Could you check a few things on this model? Use its own coordinates, in mm. A direction names the side the tool comes from. Coordinates: 2 decimals unless noted, no trailing zeros. Order: outer loops, then holes, each group sorted by start corner. A loop starts at its lowest first (then second) coordinate and runs counter-clockwise, first axis right, second up. Notation, with made-up numbers: (22.5, 16) -> (44.5, 16) arc R18 ccw to (44.5, 22) -> close; hole circle Ø10 at (16, 56.25). An arc over 180 degrees is marked (long way). Use a Markdown table: item, result. Add a question column.
1) If we section it at D-D (x = -157): Write out the boundary of the cut face in (y, z), plus the area to 3 significant figures.
2) If I drill on L1, parallel to Z at x = -50, y = 1.6; L2, parallel to Z at x = -3, y = 2.5; L3, parallel to Z at x = -130, y = 4, over which ranges is the centre line in solid material (lowest first)? Write a range as [from, to].
3) If we section it at C-C (y = -53): Write out the boundary of the cut face in (x, z), plus the area to 3 significant figures.
4) Which directions (+Z, -Z, +X, -X, +Y, -Y) give clear straight access to the entire face, cutting with the end or side of a thin tool? Please do faces 1 (the flat face through (-125, 3, 174)), 2 (the flat face through (-89, 0, 98)), 3 (the flat face through (-89, 5, 101)).
5) Will these pins go through, and if not, where does the flat tip stop? pin 1 Ø3 at (x, y) = (-146.24, -11.72) entering from -Z; pin 2 Ø5.5 at (x, y) = (-146.24, -43.28) entering from -Z; pin 3 Ø1.6 at (y, z) = (3, 120) entering from +X; pin 4 Ø12 at (x, z) = (-144.5, 20) entering from -Y.
6) If we section it at B-B (z = 73.5): Write out the boundary of the cut face in (x, y).
7) If we section it at A-A (x = -50): Write out the boundary of the cut face in (y, z), plus the area to 3 significant figures.
8) Thinking about a two-plate mould opening in Z: for faces 4 (the flat face through (-89, -27, 200)), 5 (the flat face through (0, 2, 130)), 6 (the cylindrical face through (-23.02, 1.48, 80.69)), 7 (the cylindrical face through (-42.413, 3.986, 174.168)), which applies, +Z half, -Z half, draft (parallel to the pull), parting line (faces both ways), or undercut?
Autodesk Inventor part; units mm, degrees
ref_plane "YZ Plane" through (0, 0, 0) normal (1, 0, 0) x (0, 1, 0)
ref_plane "XZ Plane" through (0, 0, 0) normal (0, 1, 0) x (-1, 0, 0)
ref_plane "XY Plane" through (0, 0, 0) normal (0, 0, 1) x (1, 0, 0)
sketch "Sketch1" plane through (0, 0, 0) normal (0, 1, 0) x (-1, 0, 0)
  line L0 (0, 0) -> (180, 0)
  line L1 (180, 0) -> (180, 200)
  line L2 (180, 200) -> (0, 200)
  line L3 (0, 200) -> (0, 0)
  circle A0 centre (130, 140) radius 35
  circle A1 centre (130, 60) radius 35
  circle A2 centre (50, 140) radius 35
  circle A3 centre (50, 60) radius 35
  line L4 (130, 140) -> (50, 140)
  line L5 (130, 140) -> (130, 60)
  circle A4 centre (130, 140) radius 34
  circle A5 centre (130, 60) radius 34
  circle A6 centre (50, 140) radius 34
  circle A7 centre (50, 60) radius 34
  point P0 (90, 140)
  point P1 (90, 200)
  point P2 (130, 100)
  point P3 (180, 100)
  dimension "d0" = 180
  dimension "d1" = 200
  dimension "d2" = 70
  dimension "d3" = 70
  dimension "d4" = 70
  dimension "d5" = 70
  dimension "d6" = 10
  dimension "d7" = 10
  dimension "d11" = 68
  dimension "d12" = 68
  dimension "d13" = 68
  dimension "d14" = 68
extrude "Extrusion1" add sketch "Sketch1" along normal blind 5 contours L3 L2 L1 L0
extrude "Extrusion2" add sketch "Sketch1" along normal blind 3 contours A0 L5 A4 L4 | A1 | A2 | L4 A4 L5 A0 | A3
sketch "Sketch2" plane through (0, 0, 200) normal (1, 0, 0) x (0, 0, -1)
  circle A0 centre (40, 2.5) radius 1
  circle A1 centre (80, 2.5) radius 1
  circle A2 centre (120, 2.5) radius 1
  circle A3 centre (160, 2.5) radius 1
  line L0 (0, 0) -> (0, 5)
  line L1 (200, 0) -> (200, 5)
  line L2 (0, 5) -> (200, 5)
  dimension "d18" = 2
  dimension "d19" = 2
  dimension "d20" = 2
  dimension "d21" = 2
  dimension "d23" = 40
  dimension "d24" = 40
  dimension "d25" = 40
  dimension "d26" = 40
  dimension "d45" = 2.5
hole "Hole1" at (0, 2.5, 40) at (0, 2.5, 80) at (0, 2.5, 120) at (0, 2.5, 160) direction (-1, 0, 0) diameter 3.242 depth 11.8
sketch "Sketch3" plane through (0, 0, 0) normal (0, -1, 0) x (1, 0, 0)
  line L0 (0, 200) -> (0, 0)
  line L1 (-180, 0) -> (-180, 200)
  line L2 (0, 200) -> (-180, 200)
  line L3 (-180, 200) -> (-180, 194)
  line L4 (-180, 194) -> (0, 194)
  line L5 (0, 194) -> (0, 200)
  dimension "d35" = 6
extrude "Extrusion3" add sketch "Sketch3" along normal blind 60
sketch "Sketch4" plane through (0, 0, 194) normal (0, 0, -1) x (-1, 0, 0)
  circle A0 centre (33.7554, -11.723) radius 5.5293
  circle A1 centre (33.7554, -43.277) radius 5.535
  circle A2 centre (146.2446, -11.723) radius 5.926
  circle A3 centre (146.2446, -43.277) radius 6.0534
  line L0 (33.7554, -11.723) -> (33.7554, -43.277)
  line L1 (33.7554, -11.723) -> (146.2446, -11.723)
  line L2 (0, 0) -> (180, 0)
  line L3 (0, -60) -> (0, 5)
  point P0 (90, -11.723)
  point P1 (90, 0)
  point P2 (33.7554, -27.5)
  point P3 (0, -27.5)
hole "Hole2" at (-33.7554, -11.723, 194) at (-33.7554, -43.277, 194) at (-146.2446, -11.723, 194) at (-146.2446, -43.277, 194) direction (0, 0, 1) diameter 4.917 depth 17.1
properties part number "LensHolder"
Answer sheet:
| question | item | result |
|---|---|---|
| 1 | outline | (-60, 194) -> (0, 194) -> (0, 160.66) -> (3, 160.66) -> (3, 162.27) -> (5, 162.27) -> (5, 200) -> (-60, 200) -> close; (0, 0) -> (5, 0) -> (5, 37.73) -> (3, 37.73) -> (3, 39.34) -> (0, 39.34) -> close; (0, 80.66) -> (3, 80.66) -> (3, 82.27) -> (5, 82.27) -> (5, 117.73) -> (3, 117.73) -> (3, 119.34) -> (0, 119.34) -> close |
| 1 | area | 934 mm2 |
| 2 | L1 | [0, 26], [94, 106], [174, 200] |
| 2 | L2 | [0, 38.38], [41.62, 78.38], [81.62, 118.38], [121.62, 158.38], [161.62, 200] |
| 2 | L3 | [0, 25], [95, 105], [175, 200] |
| 3 | outline | (-180, 194) -> (0, 194) -> (0, 200) -> (-180, 200) -> close |
| 3 | area | 1,080 mm2 |
| 4 | face 1 | +Y |
| 4 | face 2 | -Z, +X, -X, -Y |
| 4 | face 3 | +Z, -Z, +X, -X, +Y |
| 5 | pin 1 | through |
| 5 | pin 2 | z = 194 |
| 5 | pin 3 | x = -11.8 |
| 5 | pin 4 | y = 0 |
| 6 | outline | (-180, 0) -> (-161.2, 0) -> (-161.2, 3) -> (-162.29, 3) -> (-162.29, 5) -> (-180, 5) -> close; (-98.8, 0) -> (-81.2, 0) -> (-81.2, 3) -> (-82.29, 3) -> (-82.29, 5) -> (-97.71, 5) -> (-97.71, 3) -> (-98.8, 3) -> close; (-18.8, 0) -> (0, 0) -> (0, 5) -> (-17.71, 5) -> (-17.71, 3) -> (-18.8, 3) -> close |
| 7 | outline | (-60, 194) -> (0, 194) -> (0, 174) -> (3, 174) -> (3, 175) -> (5, 175) -> (5, 200) -> (-60, 200) -> close; (0, 0) -> (5, 0) -> (5, 25) -> (3, 25) -> (3, 26) -> (0, 26) -> close; (0, 94) -> (3, 94) -> (3, 95) -> (5, 95) -> (5, 105) -> (3, 105) -> (3, 106) -> (0, 106) -> close |
| 7 | area | 672 mm2 |
| 8 | face 4 | +Z half |
| 8 | face 5 | draft |
| 8 | face 6 | undercut |
| 8 | face 7 | undercut |
